The drawing under review shows one solid part. Ordinate dimensions are in mm from its lowest x, y, z. Coordinates: 2 decimals unless noted, no trailing zeros. Write each loop counter-clockwise with the first axis right and the second up, starting at its lowest first coordinate (ties: lowest second). Pieces come first, ordered by that corner, then holes. Notation, with made-up numbers: (12, 61) -> (62, 61) arc R20 ccw to (62, 99) -> close; hole circle Ø4 at (-19.75, 77.5). An arc over 180 degrees is marked (long way). One line per question, with ' | ' between items. Start each with the question number.
Q1. Wall thickness on probe 1 along Y at (x, z) = (5.25, 4.75) (1 decimal); probe 2 along X at (y, z) = (11, 3); probe 3 along Z at (x, y) = (10.5, 12) (3 decimals): over which ranges is each line inside the solid? List them lowest first.
Q2. Add section B-B on z = 1.75. State the section outline as (x, y) points.
Q3. Draft analysis for pull direction X (two halves, no side actions). For the marked faces 1, 2 and 3, state which applies: pulls with the +X half, pulls with the -X half, needs draft (parallel to the pull), parting line crosses it, or undercut.
Q4. For P1, Ø1, axis at x = 13.5, z = 3.5, coming from the +Y side; P2, Ø1, axis at y = 17, z = 4.5, coming from the +X side; P3, Ø10, axis at x = 11, y = 16, coming from the +Z side; P4, Ø4, axis at x = 3.5, z = 2.5, coming from the -Y side, all flat-tipped, find the tip position at first contact; note any pin that passes through.
Q5. Add section A-A on z = 8.25. State the section outline as (x, y) points, and give its area (3 significant figures).
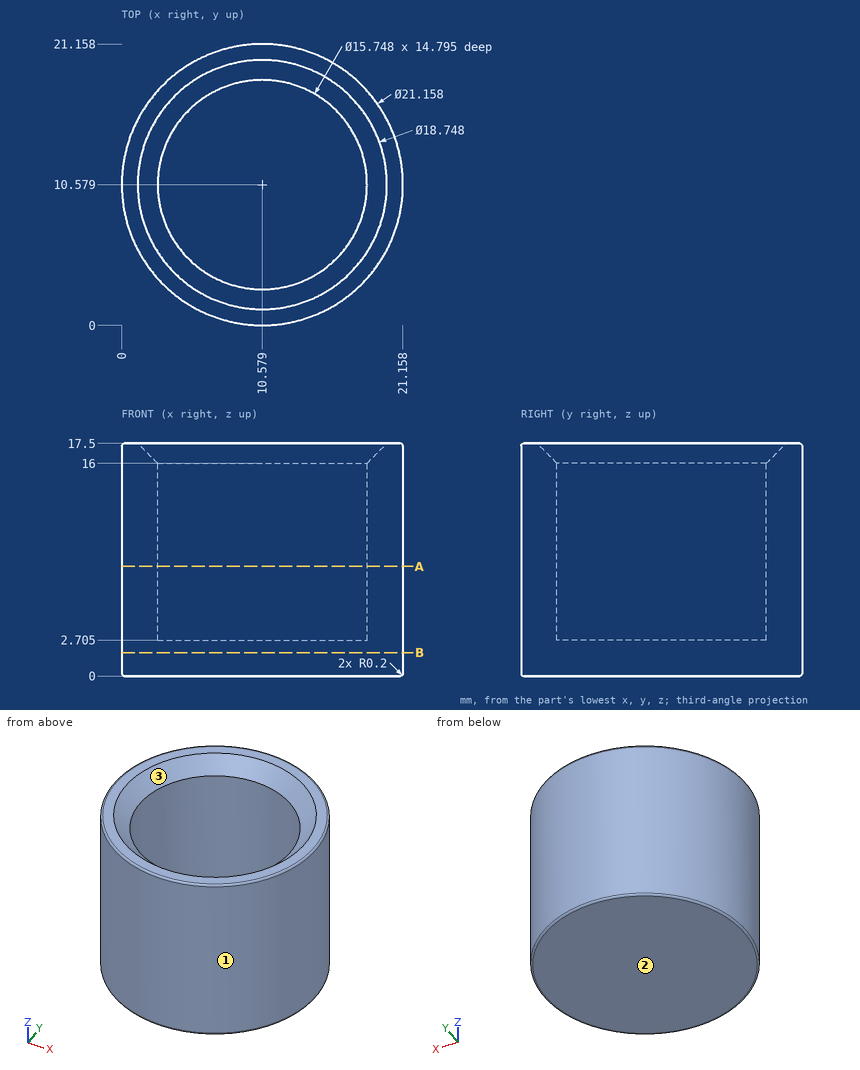
Output values:
1) probe 1: y = 1.4 to 4.8, 16.4 to 19.7 | probe 2: x = 0.01 to 2.72, 18.44 to 21.15 | probe 3: z = 0 to 2.705
2) outline: circle Ø21.16 at (10.58, 10.58)
3) face 1: parting line crosses it | face 2: needs draft | face 3: undercut
4) P1: stops at y = 20.88 | P2: stops at x = 19.35 | P3: stops at z = 17.5 | P4: stops at y = 1.3
5) outline: circle Ø21.16 at (10.58, 10.58); hole circle Ø15.75 at (10.58, 10.58) | area: 157 mm2
